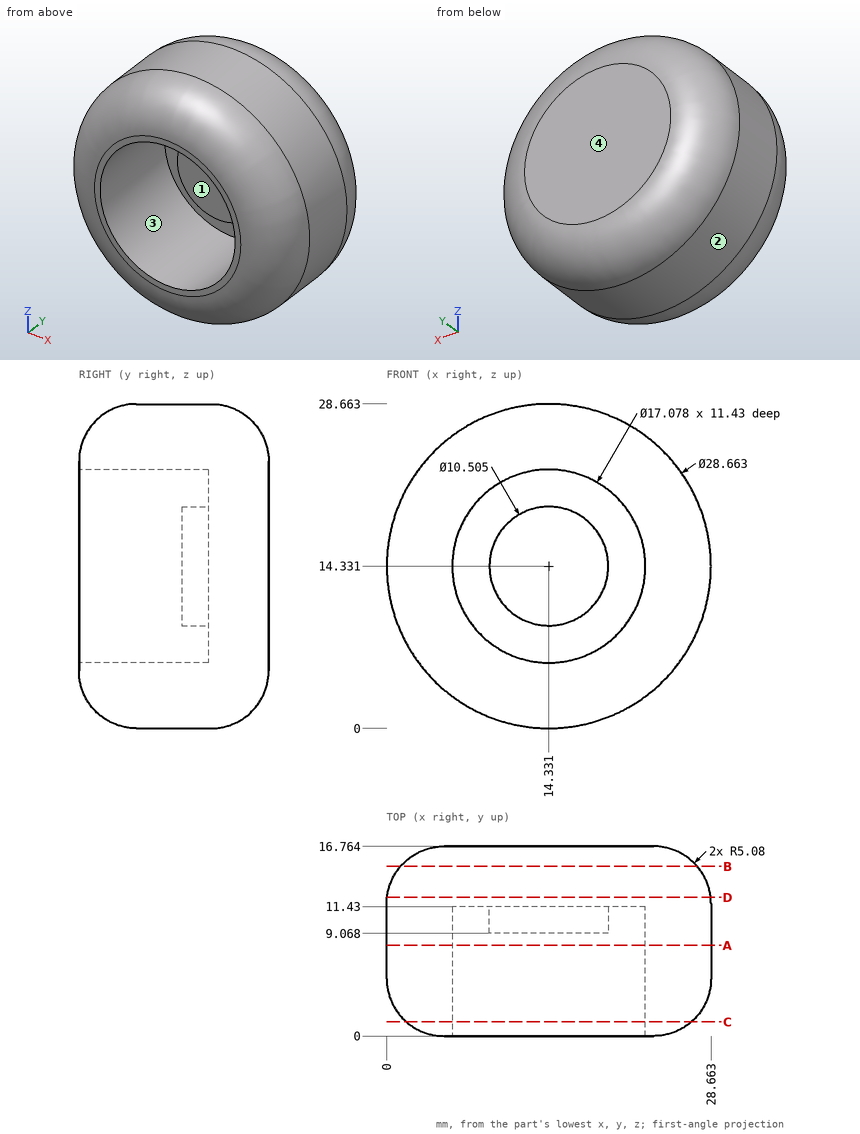
Drawing for the job (mm, zero at the part's lowest x, y, z). Give positions to 0.01 mm unless a question says otherwise; leave off trailing zeros. Loops run counter-clockwise (first coordinate to the right, second up) from the corner with the lowest first, then second, coordinate; pieces in that order, holes last. Notation, with made-up numbers: M -26.75,-20.75 L -7.75,-20.75 A31 ccw -7.75,3.25 Z; hole C 65.5,-34 d4. An arc over 180 degrees is marked long. Use one line per item in the form item = value.
Item 1: Flat gauge pins, fed straight in: pin 1 (2 mm diameter, centred on y = 3, z = 11.5, fed in from -X); pin 2 (3 mm diameter, centred on y = 14, z = 12, fed in from +X); pin 3 (4 mm diameter, centred on y = 4, z = 4.5, fed in from -X). Where does each tip first touch, or does it go through?
Determined:
pin_1 = 0.34
pin_2 = 28.47
pin_3 = 2.41
Item 2: Slice it at B-B (y = 15). List the corners of the cut face in (x, z), plus the area to 3 significant figures.
Determined:
outline = C 14.33,14.33 d26.2
area = 539 mm2
Item 3: Slice it at D-D (y = 12.25). List the corners of the cut face in (x, z), plus the area to 3 significant figures.
Determined:
outline = C 14.33,14.33 d28.6
area = 642 mm2
Item 4: Two-plate mould, pull along Z, no slides. Class the marked faces 1, 2, 3 and 4: pulls with the +Z half, pulls with the -Z half, needs draft (parallel to the pull), parting line crosses it, or undercut.
Determined:
face_1 = undercut
face_2 = parting line crosses it
face_3 = undercut
face_4 = needs draft
Item 5: Slice it at C-C (y = 1.25). List the corners of the cut face in (x, z).
Determined:
outline = C 14.33,14.33 d25.18; hole C 14.33,14.33 d17.08
Item 6: Drill centre lines: probe 1 along Z at (x, y) = (13.5, 11.25) (1 decimal); probe 2 along Y at (x, z) = (8.75, 9); probe 3 along Z at (x, y) = (16.5, 5.25) (1 decimal). Where is each one in solid material? Low to high. Write a range as from..to.
Determined:
probe_1 = 0..5.8, 9.1..19.5, 22.8..28.6
probe_2 = 11.43..16.76
probe_3 = 0.2..6.1, 22.6..28.5
Item 7: Slice it at A-A (y = 8). List the corners of the cut face in (x, z).
Determined:
outline = C 14.33,14.33 d28.66; hole C 14.33,14.33 d17.08
